CAD build for the part. Positions are in the model's coordinates, mm. Round coordinates to 2 decimals unless told otherwise and drop trailing zeros. Loops run counter-clockwise (first coordinate to the right, second up) from the corner with the lowest first, then second, coordinate; pieces in that order, holes last.
from build123d import *

# Parameters (mm, degrees)
F0_R     = 2.5
F1_DEPTH = 4


with BuildPart() as f1:
    # F0 (on Top) → F1 (new body)
    with BuildSketch(Plane.XY):
        Polygon((30, 30), (-30, 30), (-30, -30), (-10, -30), (30, 10), align=None)
        with Locations((-20, -20)):
            Circle(F0_R, mode=Mode.SUBTRACT)
        with Locations((-20, 0)):
            Circle(F0_R, mode=Mode.SUBTRACT)
        Polygon((8.786797, 10), (-10, -8.786797), (-10, 10), align=None, mode=Mode.SUBTRACT)
        with Locations((-20, 20)):
            Circle(F0_R, mode=Mode.SUBTRACT)
        with Locations((0, 20)):
            Circle(F0_R, mode=Mode.SUBTRACT)
        with Locations((20, 20)):
            Circle(F0_R, mode=Mode.SUBTRACT)
    extrude(amount=F1_DEPTH)


solid = f1.part
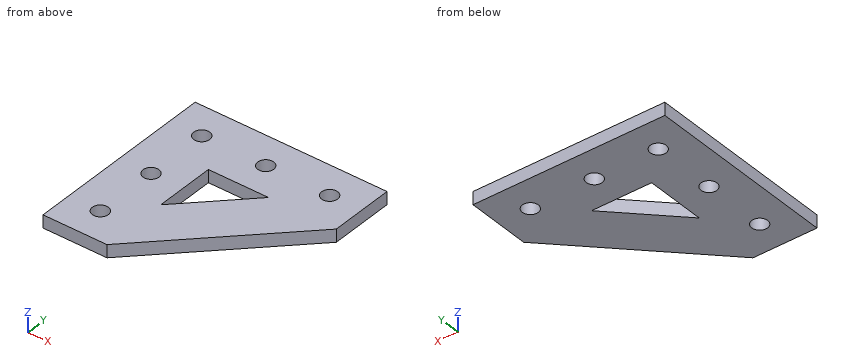
Item 1: Wall check: L1, parallel to Y at x = -20, z = 2.7; L2, parallel to X at y = 18, z = 0.55; L3, parallel to Y at x = 20, z = 3.75. Give the ranges that are in metal, low to high.
Verdict:
L1: y = -30 to -22.5, -17.5 to -2.5, 2.5 to 17.5, 22.5 to 30
L2: x = -30 to -21.5, -18.5 to -1.5, 1.5 to 18.5, 21.5 to 30
L3: y = 0 to 17.5, 22.5 to 30
Item 2: Cut at A-A (y = 20). List the corners of the cut face in (x, z).
Verdict:
outline: (-30, 0) - (-22.5, 0) - (-22.5, 4) - (-30, 4) - close; (-17.5, 0) - (-2.5, 0) - (-2.5, 4) - (-17.5, 4) - close; (2.5, 0) - (17.5, 0) - (17.5, 4) - (2.5, 4) - close; (22.5, 0) - (30, 0) - (30, 4) - (22.5, 4) - close
Item 3: Flat gauge pin, fed straight in: P1, Ø2, axis at x = 0, z = 3.5, coming from the -Y side. Where does the tip first touch, or does it go through?
Verdict:
P1: stops at y = -21
